```python
from build123d import *

# Parameters (mm, degrees)
SKETCH1_W          = 38.1
SKETCH1_H          = 25.4
SKETCH1_W_2        = 50.8
SKETCH1_H_2        = 9.525
SKETCH1_W_3        = 6.35
SKETCH1_H_3        = 41.275
FILLET1_R          = 6.35
SKETCH4_W          = 6.35
SKETCH4_H          = 15.24
CUT_EXTRUDE1_DEPTH = 51.8


with BuildPart() as part:
    # Sketch1 → Revolve1 (revolve)
    with BuildSketch(Plane(origin=(0, 0, 0), x_dir=(0, 0, -1), z_dir=(1, 0, 0))):
        with Locations((0, 76.2)):
            Rectangle(SKETCH1_W, SKETCH1_H)
        with Locations((0, 17.4625)):
            Rectangle(SKETCH1_W_2, SKETCH1_H_2)
        with Locations((0, 42.8625)):
            Rectangle(SKETCH1_W_3, SKETCH1_H_3)
    revolve(axis=Axis((0, 0, 0), (0, 0, -1)))

    # Sketch3 → Cut-Revolve1 (revolve, cut)
    with BuildSketch(Plane(origin=(0, 0, 0), x_dir=(0, 0, -1), z_dir=(1, 0, 0))):
        Polygon((-10.972421975, 88.9), (10.972421975, 88.9), (6.35, 76.2), (-6.35, 76.2), align=None)
    revolve(axis=Axis((0, 0, 0), (0, 0, -1)), mode=Mode.SUBTRACT)

    # Fillet1
    fillet1_edges = [part.edges().sort_by_distance(p)[0] for p in [
        (0, -63.5, -3.175),
        (0, -22.225, -3.175),
        (0, -22.225, 3.175),
        (0, -63.5, 3.175),
    ]]
    fillet(fillet1_edges, radius=FILLET1_R)

    # Sketch4 → Cut-Extrude1 (cut, through all)
    with BuildSketch(Plane.XY.offset(25.4)):
        with Locations((0, 7.62)):
            Rectangle(SKETCH4_W, SKETCH4_H)
    extrude(amount=-CUT_EXTRUDE1_DEPTH, mode=Mode.SUBTRACT)


solid = part.part
```
Part model, mm, in its own coordinate system. A direction names the side the tool comes from. Round coordinates to 2 decimals unless told otherwise and drop trailing zeros. Loops run counter-clockwise (first coordinate to the right, second up) from the corner with the lowest first, then second, coordinate; pieces in that order, holes last. Notation, with made-up numbers: (70, 30.25) -> (120, 30.25) arc R14 ccw to (120, 35.25) -> close; hole circle Ø7 at (43, 61). An arc over 180 degrees is marked (long way). Use a Markdown table: item, result.
1) Pull direction Y, two halves, no side cores. Call faces 5 (the cylindrical face through (-61.99, -13.77, 14.22)), 6 (the conical face through (-46.742, -60.959, -6.574)), 7 (the flat face through (21, 61, -19.05)): pulls with the +Y half, pulls with the -Y half, needs draft (parallel to the pull), parting line crosses it, or undercut.
The answers:
| item | result |
|---|---|
| face 5 | undercut |
| face 6 | parting line crosses it |
| face 7 | needs draft |
2) Drop flat-ended pins along their axis: pin 1 Ø3 at (y, z) = (13.5, 12) entering from -X; pin 2 Ø1 at (x, y) = (-5, -24) entering from +Z; pin 3 Ø5 at (x, z) = (58, 9) entering from +Y. Give the stop position or say it passes through.
The answers:
| item | result |
|---|---|
| pin 1 | stops at x = -88.09 |
| pin 2 | stops at z = 5.11 |
| pin 3 | stops at y = 68.67 |
3) Tool access for faces 1 (the cylindrical face through (18.74, 11.95, 17.35)), 2 (the cylindrical face through (18.74, 11.95, -17.57)), 3 (the flat face through (0, 15.24, 0)), 4 (the cylindrical face through (-46.367, -60.47, 0.089)): list every direction of +Z, -Z, +X, -X, +Y, -Y with a clear straight run to the whole face (end or side of a thin tool).
The answers:
| item | result |
|---|---|
| face 1 | +Z |
| face 2 | -Z |
| face 3 | +Z, -Z |
| face 4 | none |
4) Cut at B-B, the plane z = 0. List the corners of the cut face in (x, y) (3 decimals).
The answers:
| item | result |
|---|---|
| outline | circle Ø152.4 at (0, 0); hole (-3.175, 12.297) arc R12.7 ccw (long way) to (3.175, 12.297) -> (3.175, 15.24) -> (-3.175, 15.24) -> close |
5) Cut at A-A, the plane z = 14.5. List the corners of the cut face in (x, y) (3 decimals), and give its area (3 significant figures).
The answers:
| item | result |
|---|---|
| outline | circle Ø177.8 at (0, 0); circle Ø44.45 at (0, 0); hole circle Ø127 at (0, 0); hole (-3.175, 12.297) arc R12.7 ccw (long way) to (3.175, 12.297) -> (3.175, 15.24) -> (-3.175, 15.24) -> close |
| area | 13,200 mm2 |
6) Probe line 1 (X direction, y = 0, z = -15) (3 decimals); line 2 (X direction, y = 0, z = -3); line 3 (Y direction, x = 16, z = -12.5). List the from-to ranges inside material, lowest first. Write a range as [from, to].
The answers:
| item | result |
|---|---|
| line 1 | x = [-88.9, -63.5], [-22.225, -12.7], [12.7, 22.225], [63.5, 88.9] |
| line 2 | x = [-76.2, -12.7], [12.7, 76.2] |
| line 3 | y = [-87.45, -61.45], [-15.43, 15.43], [61.45, 87.45] |
